Can you work these out from the model? Positions are in its coordinate system, mm. A direction names the side the tool comes from. Give positions to 0.01 mm unless a question says otherwise; leave off trailing zeros. Loops run counter-clockwise (first coordinate to the right, second up) from the corner with the lowest first, then second, coordinate; pieces in that order, holes last. Notation, with made-up numbers: (59.5, -37.5) - (113.5, -37.5) arc R6 cw to (113.5, -27.5) - close; hole circle Ø8 at (-11.75, 68.5). An arc over 180 degrees is marked (long way). Write item = value, one per line.
from build123d import *

# Parameters (mm, degrees)
F1_DEPTH       = 16
F2_W           = 70
F2_H           = 3
F3_DEPTH       = 2
F4_W           = 50
F4_H           = 14
F5_DEPTH       = 2
F6_R           = 1
F9_DEPTH       = 2
F11_DEPTH      = 21.001
F11_DEPTH_BACK = 25
F13_D          = 4
F14_W          = 50
F14_H          = 11
F14_R          = 3
F15_DEPTH      = 5
F16_R          = 3


# Not quite as in the source:
# - a pattern or mirror of a feature is missing from the dataset's text; its kind, count and spacing are read off the source's solid


with BuildPart() as f1:
    # F0 (on Front) → F1 (new body)
    with BuildSketch(Plane.XZ):
        with BuildLine():
            ThreePointArc((0, -9), (-9, 0), (0, 9))
            Line((0, 9), (94, 9))
            Line((94, 9), (94, 11))
            Line((94, 11), (0, 11))
            ThreePointArc((0, 11), (-11, 0), (0, -11))
            Line((0, -11), (19, -11))
            ThreePointArc((19, -11), (21.7681124643, -11.8361612201), (23.6103896104, -14.064978646))
            ThreePointArc((23.6103896104, -14.064978646), (52.3002338891, -47.5417473959), (95.1260447976, -58.0179647813))
            ThreePointArc((95.1260447976, -58.0179647813), (99.0798371754, -59.7246197028), (102.3278575446, -62.552252789))
            Line((102.3278575446, -62.552252789), (103.6303522873, -61))
            ThreePointArc((103.6303522873, -61), (99.852279938, -57.8519370421), (95.2965735981, -56))
            ThreePointArc((95.2965735981, -56), (53.4811996085, -45.9198240056), (25.4545454545, -13.2909701044))
            ThreePointArc((25.4545454545, -13.2909701044), (22.87535745, -10.1706257081), (19, -9))
            Line((19, -9), (0, -9))
        make_face()
    extrude(amount=F1_DEPTH)

    # F2 (on face) → F3 (join)
    with BuildSketch(Plane.XY.offset(11)):
        with Locations((59, -17.5)):
            Rectangle(F2_W, F2_H)
    extrude(amount=-F3_DEPTH)

    # F4 (on face) → F5 (join)
    with BuildSketch(Plane.XZ.offset(19)):
        with Locations((69, 4)):
            Rectangle(F4_W, F4_H)
    extrude(amount=F5_DEPTH)

    # F6
    f6_edges = [f1.edges().sort_by_distance(p)[0] for p in [
        (69, -21, 11),
        (69, -19, 9),
    ]]
    fillet(f6_edges, radius=F6_R)

    # F7: F1 across plane


with BuildPart() as f1_1:
    add(f1.part)
    add(f1.part.mirror(Plane.XZ))

    # F8 (on face) → F9 (cut)
    with BuildSketch(Plane.XY.offset(11)):
        with BuildLine():
            Line((94, 12), (34, 12))
            ThreePointArc((34, 12), (22, 0), (34, -12))
            Line((34, -12), (94, -12))
            Line((94, -12), (94, 12))
        make_face()
    extrude(amount=-F9_DEPTH, mode=Mode.SUBTRACT)

    # F10 (on Front) → F11 (cut, two sides)
    with BuildSketch(Plane.XZ) as f11_sk:
        with BuildLine():
            ThreePointArc((50, 5), (47, 2), (50, -1))
            Line((50, -1), (70, -1))
            ThreePointArc((70, -1), (73, 2), (70, 5))
            Line((70, 5), (50, 5))
        make_face()
    extrude(amount=-F11_DEPTH, mode=Mode.SUBTRACT)
    extrude(f11_sk.sketch, amount=F11_DEPTH_BACK, mode=Mode.SUBTRACT)

    # F13 (through all)
    with Locations(Plane.XZ.offset(21)):
        with Locations((80, 2)):
            Hole(F13_D / 2)

    # F14 (on face) → F15 (join)
    with BuildSketch(Plane(origin=(0, -19, 0), x_dir=(-1, 0, 0), z_dir=(0, 1, 0))):
        with Locations((-69, 2.5)):
            Rectangle(F14_W, F14_H)
        with Locations((-80, 2)):
            Circle(F14_R, mode=Mode.SUBTRACT)
        with BuildLine():
            Line((-70, 5), (-50, 5))
            ThreePointArc((-50, 5), (-47, 2), (-50, -1))
            Line((-50, -1), (-70, -1))
            ThreePointArc((-70, -1), (-73, 2), (-70, 5))
        make_face(mode=Mode.SUBTRACT)
    f15 = extrude(amount=F15_DEPTH)

    # F15_copies: F15 across plane
    add(f15.mirror(Plane.ZX))

    # F16
    f16_edges = [f1_1.edges().sort_by_distance(p)[0] for p in [
        (44, -17.5, -3),
        (94, -17.5, -3),
        (44, 17.5, -3),
        (94, 17.5, -3),
    ]]
    fillet(f16_edges, radius=F16_R)


solid = f1_1.part
Q1. We'd pull the mould along X, two halves only. Please class faces 1 (the flat face through (94, -18, 5)), 2 (the cylindrical face through (44.86, 17.55, -2.1)), 3 (the flat face through (10, 0, -9)): released by +X, released by -X, zero draft, split by the parting line, or undercut.
Output:
face_1 = released by +X
face_2 = undercut
face_3 = zero draft
Q2. Imagine slicing it at B-B, the plane x = 66. Give the number of separate pieces and of enclosed holes in the cut face, then the cut area to 3 significant figures.
Output:
separate_pieces = 5
enclosed_holes = 0
area = 178 mm2
Q3. Which directions (+Z, -Z, +X, -X, +Y, -Y) give clear straight access to the entire face, cutting with the end or side of a thin tool? Please do faces 4 (the flat face through (60, -18, 5)), 5 (the flat face through (9, 0, -11)), 6 (the flat face through (75, -14, 3)).
Output:
face_4 = +Y, -Y
face_5 = -Z, -X, +Y, -Y
face_6 = +X
Q4. I need wall thicknesses on L1, parallel to Z at x = 80, y = -17.35; L2, parallel to Z at x = 68, y = -14.5; L3, parallel to Z at x = 80, y = -15. Which ranges of each line are inside material? Lowest first, please.
Output:
L1 = -3 to -1, 5 to 8, 9 to 11
L2 = -54.76 to -52.65, -3 to -1, 5 to 8, 9 to 11
L3 = -57.5 to -55.48, -3 to -1, 5 to 8, 9 to 11
Q5. Imagine slicing it at A-A, the plane x = 38.5. Write out the boundary of the cut face in (y, z), then the cut area to 3 significant figures.
Output:
outline = (-19, 9) - (-12, 9) - (-12, 11) - (-19, 11) - close; (-16, -36.52) - (16, -36.52) - (16, -33.61) - (-16, -33.61) - close; (12, 9) - (19, 9) - (19, 11) - (12, 11) - close
area = 121 mm2
Q6. Imagine slicing it at D-D, the plane y = -8.5. Write out the boundary of the cut face in (x, z), then the cut area to 3 significant figures.
Output:
outline = (0, -11) - (19, -11) arc R5 cw to (23.61, -14.06) arc R72 ccw to (95.13, -58.02) arc R14 cw to (102.33, -62.55) - (103.63, -61) arc R16 ccw to (95.3, -56) arc R70 cw to (25.45, -13.29) arc R7 ccw to (19, -9) - (0, -9) arc R9 cw to (0, 9) - (25.53, 9) - (25.53, 11) - (0, 11) arc R11 ccw to start
area = 362 mm2
Q7. For pin 1 (10 mm diameter, centred on x = 44, y = -2, fed in from -Z); pin 2 (10 mm diameter, centred on x = 32, y = 4.5, fed in from -Z); pin 3 (7 mm diameter, centred on y = 18.5, z = 7, fed in from +X), each with a flat end and sliding along its axis, tell me the tip position at first contact or that it passes through.
Output:
pin_1 = -45.39
pin_2 = -34.93
pin_3 = 94
